Could you check a few things on this drawing? It's one solid part, dimensions in mm from its lowest x, y, z. A direction names the side the tool comes from. Give positions to 0.01 mm unless a question says otherwise; leave off trailing zeros. Loops run counter-clockwise (first coordinate to the right, second up) from the corner with the lowest first, then second, coordinate; pieces in that order, holes last. Notation, with made-up numbers: M -27,85.5 L 10,85.5 A23 ccw 10,115.5 Z; hole C 2.25,-1.75 d9. An arc over 180 degrees is marked long. Answer in a Markdown table with one row per item. Add a question column.
1. If we section it at A-A on y = 18: List the corners of the cut face in (x, z) for me.
2. If we section it at D-D on z = 10.5: List the corners of the cut face in (x, y) for me, then the cut area to 3 significant figures.
3. I need wall thicknesses on line 1 along X through (y, z) = (28, 11); line 2 along Y through (x, z) = (41, 7.5); line 3 along Z through (x, y) = (49, 75). Which ranges of each line are inside material? Lowest first, please. Write a range as from..to.
4. If we section it at B-B on x = 17.5: List the corners of the cut face in (y, z) for me, then the cut area to 3 significant figures.
5. Which directions (+Z, -Z, +X, -X, +Y, -Y) give clear straight access to the entire face, cutting with the end or side of a thin tool? Please do the marked faces 5 and 6.
6. Thinking about a two-plate mould opening in Y: for the marked faces 1, 2, 3 and 4, which applies, released by +Y, released by -Y, zero draft, split by the parting line, or undercut?
7. I'm going to push flat-ended pins straight in: pin 1 Ø1.5 at (x, z) = (26, 5) entering from +Y; pin 2 Ø7 at (x, y) = (26, 75) entering from +Z; pin 3 Ø1 at (x, y) = (9, 58) entering from +Z. Where does each tip first touch, or does it pass through?
8. If we section it at C-C on z = 15.5: List the corners of the cut face in (x, y) for me, then the cut area to 3 significant figures.
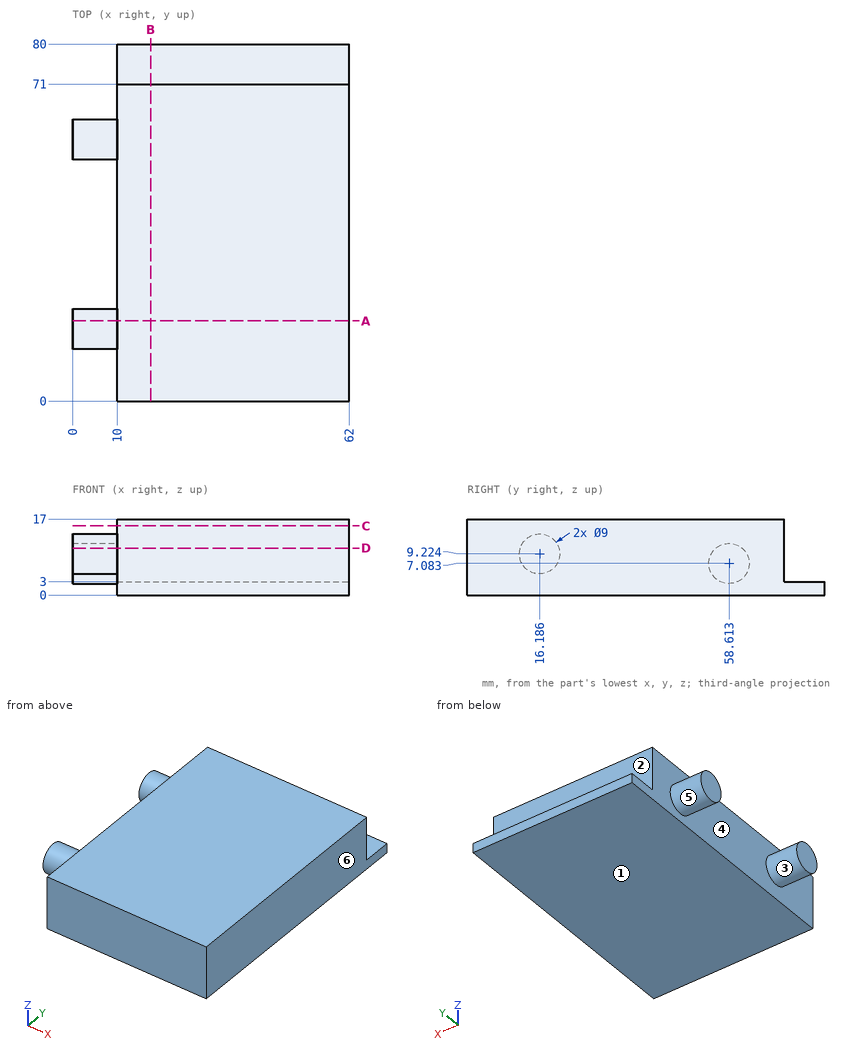
Results:
| question | item | result |
|---|---|---|
| 1 | outline | M 0,5.11 L 10,5.11 L 10,0 L 62,0 L 62,17 L 10,17 L 10,13.34 L 0,13.34 Z |
| 2 | outline | M 0,11.87 L 10,11.87 L 10,0 L 62,0 L 62,71 L 10,71 L 10,61.54 L 0,61.54 L 0,55.68 L 10,55.68 L 10,20.5 L 0,20.5 Z |
| 2 | area | 3,840 mm2 |
| 3 | line 1 | 10..62 |
| 3 | line 2 | 0..71 |
| 3 | line 3 | 0..3 |
| 4 | outline | M 0,0 L 80,0 L 80,3 L 71,3 L 71,17 L 0,17 Z |
| 4 | area | 1,230 mm2 |
| 5 | face 5 | -X |
| 5 | face 6 | +Z, -Z, +X, +Y, -Y |
| 6 | face 1 | zero draft |
| 6 | face 2 | released by +Y |
| 6 | face 3 | undercut |
| 6 | face 4 | undercut |
| 7 | pin 1 | y = 71 |
| 7 | pin 2 | z = 3 |
| 7 | pin 3 | z = 11.58 |
| 8 | outline | M 10,0 L 62,0 L 62,71 L 10,71 Z |
| 8 | area | 3,690 mm2 |
